CAD build for the part. Positions are in the model's coordinates, mm. Face numbers are marked on the shaded views. Give positions to 0.01 mm unless a question says otherwise; leave off trailing zeros. Write each loop counter-clockwise with the first axis right and the second up, starting at its lowest first coordinate (ties: lowest second). Pieces come first, ordered by that corner, then holes. Notation, with made-up numbers: (-2, -8.75) - (48, -8.75) arc R26 cw to (48, 19.25) - close; hole circle Ø6 at (-34.5, -20.75). An arc over 180 degrees is marked (long way). Put each result on its own line as item: value. Start each with the question number.
1. Cut at B-B on y = 3. List the corners of the cut face in (x, z), and give its area (3 significant figures).
2. Cut at A-A on z = 0. List the corners of the cut face in (x, y).
3. Wall check: line 1 (X direction, y = -4.75, z = 0); line 2 (X direction, y = 1.5, z = 0.75). Give the ranges that are in metal, low to high.
4. Mould opens along X. For the marked faces 1, 2 and 3 say: +X half, -X half, draft (parallel to the pull), parting line (faces both ways), or undercut.
5. Cut at C-C on y = 1.25. List the corners of the cut face in (x, z) (3 decimals).
6. Drop flat-ended pins along their axis: pin 1 (2 mm diameter, centred on x = 3.5, y = -4, fed in from -Z); pin 2 (1 mm diameter, centred on x = -4.5, y = -2, fed in from +Z); pin 3 (6 mm diameter, centred on y = -3.5, z = -1.5, fed in from +X). Give the stop position or say it passes through.
from build123d import *

# Parameters (mm, degrees)
CROQUIS3_R              = 6.25
CROQUIS3_R_2            = 4.25
SALIENTE_EXTRUIR1_DEPTH = 7.5
CORTAR_EXTRUIR1_DEPTH   = 10


with BuildPart() as part:
    # Croquis2 → Revolución1 (revolve)
    with BuildSketch(Plane.XY):
        Polygon((-4.25, 0), (-8, 7.5), (-10, 7.5), (-6.25, 0), align=None)
    revolve(axis=Axis((0, 7.5, 0), (0, -1, 0)))

    # Croquis3 → Saliente-Extruir1 (add)
    with BuildSketch(Plane.XZ):
        Circle(CROQUIS3_R)
        Circle(CROQUIS3_R_2, mode=Mode.SUBTRACT)
    extrude(amount=SALIENTE_EXTRUIR1_DEPTH)

    # Croquis4 → Cortar-Extruir1 (cut)
    with BuildSketch(Plane(origin=(0, 7.5, 0), x_dir=(1, 0, 0), z_dir=(0, 1, 0))):
        Polygon((-7.816541924, 8), (7.816541924, 8), (0, 11.458627945), align=None)
    extrude(amount=-CORTAR_EXTRUIR1_DEPTH, mode=Mode.SUBTRACT)


solid = part.part
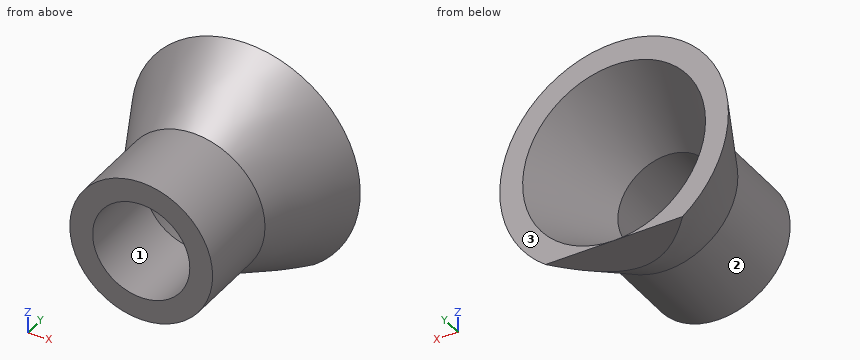
Report:
1. outline: circle Ø15.5 at (0, 0); hole circle Ø11.5 at (0, 0)
1. area: 84.8 mm²
2. outline: (-10, 7.5) - (-6.25, 0) - (-6.25, -7.5) - (-4.25, -7.5) - (-4.25, 0) - (-8, 7.5) - close; (4.25, -7.5) - (6.25, -7.5) - (6.25, 0) - (10, 7.5) - (8, 7.5) - (4.25, 0) - close
3. line 1: x = -6.25 to -4.25, 4.25 to 6.25
3. line 2: x = -6.96 to -4.94, 4.94 to 6.96
4. face 1: undercut
4. face 2: parting line
4. face 3: draft
5. outline: circle Ø13.75 at (0, 0); hole circle Ø9.75 at (0, 0)
6. pin 1: stops at z = -5.73
6. pin 2: stops at z = 4.8
6. pin 3: stops at x = 6.25
